Input: part model. Units: mm. Frame: model coordinates. Coordinates: 2 decimals unless noted, no trailing zeros. Order: outer loops, then holes, each group sorted by start corner. A loop starts at its lowest first (then second) coordinate and runs counter-clockwise, first axis right, second up. Notation, with made-up numbers: (48.25, 87) -> (102.25, 87) arc R19 cw to (102.25, 112) -> close; hole circle Ø8 at (10.25, 55.5). An arc over 180 degrees is marked (long way). Use one line per item in the form item = value. Start each with the question number.
1) Section query B-B on x = -2.25. Output: boundary loops of the cut face in (y, z), then the cut area to 3 significant figures.
2) Draft query along Y for faces 1 (the cylindrical face through (-0.33, 2.52, -15.65)), 2 (the flat face through (1.96, -3.34, -15.65)), 3 (the flat face through (-2, -2, 0)). Return one class per face: pulls with the +Y half, pulls with the -Y half, needs draft (parallel to the pull), parting line crosses it, or undercut.
3) Ray query, line 1 along X through (y, z) = (0.5, -10); line 2 along X through (y, z) = (1.5, -14); line 3 along Y through (x, z) = (-1, -6). Return the intervals inside material, ascending.
4) Section query C-C on z = -26. Output: boundary loops of the cut face in (x, y), then the cut area to 3 significant figures.
5) Pin query (flat end, axial travel): pin 1 (1 mm diameter, centred on x = -0.5, y = -1.5, fed in from -Z); pin 2 (1 mm diameter, centred on y = -3, z = -4.5, fed in from -X); pin 3 (3 mm diameter, centred on x = 2, z = -24.5, fed in from +Y); pin 4 (3 mm diameter, centred on x = 1, z = -28.5, fed in from -Y). Return the tip coordinate at first contact, or that it passes through.
6) Section query A-A on y = 0. Output: boundary loops of the cut face in (x, z).
Autodesk Inventor part; units mm, degrees
ref_plane "YZ Plane" through (0, 0, 0) normal (1, 0, 0) x (0, 1, 0)
ref_plane "XZ Plane" through (0, 0, 0) normal (0, 1, 0) x (-1, 0, 0)
ref_plane "XY Plane" through (0, 0, 0) normal (0, 0, 1) x (1, 0, 0)
sketch "Sketch1" plane through (0, 0, 0) normal (0, 0, 1) x (1, 0, 0)
  circle A0 centre (0, 0) radius 3.81
  circle A1 centre (0, 0) radius 2.54
  line L0 (0, 4.4715) -> (3.8725, 2.2358)
  line L1 (3.8725, 2.2358) -> (3.8725, -2.2358)
  line L2 (3.8725, -2.2358) -> (0, -4.4715)
  line L3 (0, -4.4715) -> (-3.8725, -2.2358)
  line L4 (-3.8725, -2.2358) -> (-3.8725, 2.2358)
  line L5 (-3.8725, 2.2358) -> (0, 4.4715)
  dimension "d0" = 5.08
  dimension "d1" = 7.62
extrude "Extrusion1" add sketch "Sketch1" against normal blind 31.75 contours A0 | L0 L1 L2 L3 L4 L5
properties part number "Stand offs BD motor mount"
Answers below:
q1.outline = (-3.17, -31.75) -> (-1.18, -31.75) -> (-1.18, 0) -> (-3.17, 0) -> close; (1.18, -31.75) -> (3.17, -31.75) -> (3.17, 0) -> (1.18, 0) -> close
q1.area = 127 mm^2
q2.face_1 = undercut
q2.face_2 = pulls with the -Y half
q2.face_3 = needs draft
q3.line_1 = -3.87 to -2.49, 2.49 to 3.87
q3.line_2 = -3.87 to -2.05, 2.05 to 3.87
q3.line_3 = -3.89 to -2.33, 2.33 to 3.89
q4.outline = (-3.87, -2.24) -> (0, -4.47) -> (3.87, -2.24) -> (3.87, 2.24) -> (0, 4.47) -> (-3.87, 2.24) -> close; hole circle Ø5.08 at (0, 0)
q4.area = 31.7 mm^2
q5.pin_1 = through
q5.pin_2 = -3.41
q5.pin_3 = 4.18
q5.pin_4 = -4.47
q6.outline = (-3.87, -31.75) -> (-2.54, -31.75) -> (-2.54, 0) -> (-3.87, 0) -> close; (2.54, -31.75) -> (3.87, -31.75) -> (3.87, 0) -> (2.54, 0) -> close
